Geometry: final body of the model. Coordinates: model frame, mm. Give positions to 0.01 mm unless a question says otherwise; leave off trailing zeros. Write each loop counter-clockwise with the first axis right and the second up, starting at its lowest first coordinate (ties: lowest second). Pieces come first, ordered by that corner, then holes.
Q1. Section C-C (z = 122). Return the cut outline in (x, y), plus the area to 3 significant figures.
Q2. Pin query (flat end, axial travel): pin 1 Ø15 at (x, y) = (-113.5, 218) entering from -Z. Return the tip coordinate at first contact, or that it passes through.
Q3. Section B-B (z = 234). Return the cut outline in (x, y).
Q4. Section A-A (y = 241). Return the cut outline in (x, z), plus the area to 3 significant figures.
Q5. Line query: line 1 (Z direction, x = -82, y = 245.5); line 2 (X direction, y = 236, z = 122); line 3 (X direction, y = 248, z = 76.5). Output: solid intervals per line, ascending.
from build123d import *

# Parameters (mm, degrees)
F4_DEPTH = 50


with BuildPart() as f4:
    # F3 (on plane+point) → F4 (new body)
    with BuildSketch(Plane.XZ.offset(-255)):
        Polygon((-152.5, 265.7889200098), (-47.5, 265.7889200098), (-8.9356621785, 50), (1048.9356621785, 50), (1087.5, 265.7889200098), (1192.5, 265.7889200098), (1192.5, 475.7889200098), (-152.5, 475.7889200098), align=None)
    extrude(amount=F4_DEPTH)


solid = f4.part
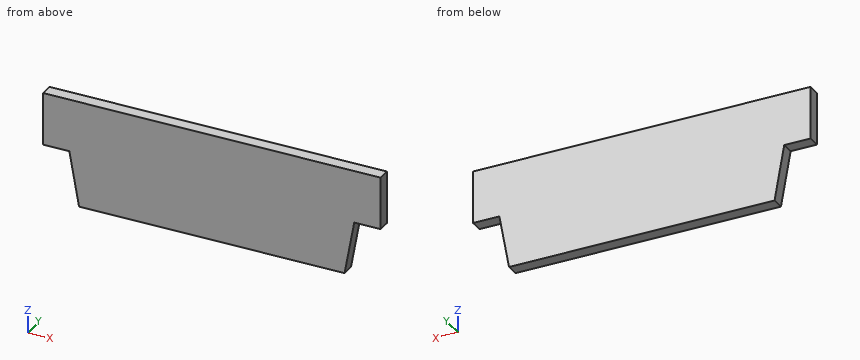
Computed:
1. outline: (-21.8, 205) - (1061.8, 205) - (1061.8, 255) - (-21.8, 255) - close
1. area: 54,200 mm2
2. pin 1: stops at z = 265.79
3. outline: (-41.82, 205) - (1081.82, 205) - (1081.82, 255) - (-41.82, 255) - close
4. outline: (-152.5, 265.79) - (-47.5, 265.79) - (-8.94, 50) - (1048.94, 50) - (1087.5, 265.79) - (1192.5, 265.79) - (1192.5, 475.79) - (-152.5, 475.79) - close
4. area: 519,000 mm2
5. line 1: z = 265.79 to 475.79
5. line 2: x = -21.8 to 1061.8
5. line 3: x = -13.67 to 1053.67
